The model under review builds one solid part; all positions refer to its coordinate system, in mm. A direction names the side the tool comes from. Coordinates: 2 decimals unless noted, no trailing zeros. Loops run counter-clockwise (first coordinate to the right, second up) from the corner with the lowest first, then second, coordinate; pieces in that order, holes last. Notation, with made-up numbers: (-34, -12.5) - (23, -12.5) arc R13 ccw to (23, -7.5) - close; hole circle Ø1 at (75.25, -3.5). An arc over 180 degrees is marked (long way). Answer in a Markdown table with one row per item. Add a question column.
(1) We need section A-A on x = -38.1. Write out the cut boundary in (y, z), plus the area to 3 significant figures.
(2) We need section B-B on y = 12.7. Write out the cut boundary in (x, z), plus the area to 3 significant figures.
(3) We need section C-C on y = 0. Give the number of separate pieces and of enclosed holes in the cut face, plus the area to 3 significant figures.
(4) For P1, Ø0.8, axis at y = -16.5, z = 0.5, coming from the +X side; P2, Ø2.5, axis at x = -62.5, y = -2, coming from the +Z side; P3, Ø0.6, axis at x = -65.5, z = 0, coming from the -Y side; P4, Ø0.8, axis at y = -7.5, z = 0, coming from the +X side, all flat-tipped, find the tip position at first contact; note any pin that passes through.
(5) Mouldability with a two-part tool opening along Y and no side actions: class faces 3 (the flat face through (-1, 38.1, 9)), 4 (the flat face through (-1, -38.1, 9)), 5 (the cylindrical face through (63, -15.293, 1.198)) as +Y half, -Y half, draft (parallel to the pull), parting line (faces both ways), or undercut.
(6) For line 1 along X through (y, z) = (-12.7, 13.75); line 2 along X through (y, z) = (11, 8.75); line 3 along Y through (x, z) = (63.5, 9.25), list the stretches that pass through material, from the lowest coordinate up.
(7) Machinability: for faces 1 (the cylindrical face through (58.25, -15.04, 9.46)), 2 (the flat face through (68.67, -31.66, 8.96)), which of the approach directions +Z, -Z, +X, -X, +Y, -Y give a long, thin tool a straight path to every point of the face, cutting with its end or side? Answer none if there is none.
from build123d import *

# Parameters (mm, degrees)
SKETCH1_W                                    = 149.86
SKETCH1_H                                    = 76.2
EXTRUDE1_DEPTH                               = 17.399
SKETCH2_W                                    = 149.86
SKETCH2_H                                    = 76.2
SKETCH2_W_2                                  = 19.05
SKETCH2_H_2                                  = 38.1
CUT_EXTRUDE1_DEPTH                           = 0.762
F_10_32_TAPPED_HOLE1_D                       = 4.0386
CBORE_FOR_10_SOCKET_HEAD_CAP_SCREW1_AT_COUNT = 2
CBORE_FOR_10_SOCKET_HEAD_CAP_SCREW1_AT_PITCH = 25.4
CBORE_FOR_10_SOCKET_HEAD_CAP_SCREW1_2_COUNT  = 2
CBORE_FOR_10_SOCKET_HEAD_CAP_SCREW1_2_PITCH  = 124.499845703
CHAMFER1_SIZE                                = 12.7
SKETCH7_W                                    = 1.5748
SKETCH7_H                                    = 38.1
CUT_EXTRUDE2_DEPTH                           = 0.762
F_13_32_0_40625_DIAMETER_HOLE1_D             = 10.31875


with BuildPart() as part:
    # Sketch1 → Extrude1 (new body)
    with BuildSketch(Plane.XY):
        Rectangle(SKETCH1_W, SKETCH1_H)
    extrude(amount=EXTRUDE1_DEPTH)

    # Sketch2 → Cut-Extrude1 (cut)
    with BuildSketch(Plane(origin=(0, 0, 0), x_dir=(-1, 0, 0), z_dir=(0, 0, -1))):
        Rectangle(SKETCH2_W, SKETCH2_H)
        with Locations((-61.9252, 0)):
            Rectangle(SKETCH2_W_2, SKETCH2_H_2, mode=Mode.SUBTRACT)
        with Locations((61.9252, 0)):
            Rectangle(SKETCH2_W_2, SKETCH2_H_2, mode=Mode.SUBTRACT)
    extrude(amount=-CUT_EXTRUDE1_DEPTH, mode=Mode.SUBTRACT)

    # #10-32 Tapped Hole1 (through all)
    with Locations(Plane.XY.offset(17.399)):
        with Locations((61.9252, 0), (-61.9252, -12.7), (-61.9252, 12.7)):
            Hole(F_10_32_TAPPED_HOLE1_D / 2)

    # Sketch5 → CBORE for #10 Socket Head Cap Screw1 (revolve, cut)
    with BuildSketch(Plane(origin=(61.9252, -12.7, 17.399), x_dir=(0, -1, 0), z_dir=(1, 0, 0))):
        Polygon((0, 0), (0, 17.399), (2.8067, 17.399), (2.8067, 15.0368), (4.3561, 15.0368), (4.3561, 1.0414), (5.3975, 0), align=None)
    cbore_for_10_socket_head_cap_screw1 = revolve(axis=Axis((61.9252, -12.7, 23.749), (0, 0, -1)), mode=Mode.SUBTRACT)

    # CBORE for #10 Socket Head Cap Screw1 at: CBORE for #10 Socket Head Cap Screw1 ×2
    with Locations(*[(0, i * CBORE_FOR_10_SOCKET_HEAD_CAP_SCREW1_AT_PITCH, 0) for i in range(1, CBORE_FOR_10_SOCKET_HEAD_CAP_SCREW1_AT_COUNT)]):
        add(cbore_for_10_socket_head_cap_screw1, mode=Mode.SUBTRACT)

    # CBORE for _10 Socket Head Cap Screw1 2: CBORE for #10 Socket Head Cap Screw1 ×2
    with Locations(*[Vector(-0.994783562, 0.102008159, 0) * (i * CBORE_FOR_10_SOCKET_HEAD_CAP_SCREW1_2_PITCH) for i in range(1, CBORE_FOR_10_SOCKET_HEAD_CAP_SCREW1_2_COUNT)]):
        add(cbore_for_10_socket_head_cap_screw1, mode=Mode.SUBTRACT)

    # Chamfer1
    chamfer1_edges = [part.edges().sort_by_distance(p)[0] for p in [
        (74.93, -38.1, 9.0805),
        (-74.93, -38.1, 9.0805),
        (-74.93, 38.1, 9.0805),
        (74.93, 38.1, 9.0805),
    ]]
    chamfer(chamfer1_edges, length=CHAMFER1_SIZE)

    # Sketch7 → Cut-Extrude2 (cut)
    with BuildSketch(Plane(origin=(0, 0, 0), x_dir=(-1, 0, 0), z_dir=(0, 0, -1))):
        with Locations((61.9252, 0)):
            Rectangle(SKETCH7_W, SKETCH7_H)
        with Locations((-61.9252, 0)):
            Rectangle(SKETCH7_W, SKETCH7_H)
    extrude(amount=-CUT_EXTRUDE2_DEPTH, mode=Mode.SUBTRACT)

    # 13/32 (0.40625) Diameter Hole1 (through all)
    with Locations(Plane.XY.offset(17.399)):
        with Locations((-38.1, 0), (38.1, 0)):
            Hole(F_13_32_0_40625_DIAMETER_HOLE1_D / 2)


solid = part.part
Outcome:
| question | item | result |
|---|---|---|
| 1 | outline | (-38.1, 0.76) - (-5.16, 0.76) - (-5.16, 17.4) - (-38.1, 17.4) - close; (5.16, 0.76) - (38.1, 0.76) - (38.1, 17.4) - (5.16, 17.4) - close |
| 1 | area | 1,100 mm² |
| 2 | outline | (-74.93, 0.76) - (-71.45, 0.76) - (-71.45, 0) - (-63.94, 0) - (-63.94, 17.4) - (-74.93, 17.4) - close; (-59.91, 0) - (-52.4, 0) - (-52.4, 0.76) - (52.4, 0.76) - (52.4, 0) - (59.12, 0) - (59.12, 2.36) - (57.57, 2.36) - (57.57, 16.36) - (56.53, 17.4) - (-59.91, 17.4) - close; (64.73, 0) - (71.45, 0) - (71.45, 0.76) - (74.93, 0.76) - (74.93, 17.4) - (67.32, 17.4) - (66.28, 16.36) - (66.28, 2.36) - (64.73, 2.36) - close |
| 2 | area | 2,310 mm² |
| 3 | separate pieces | 5 |
| 3 | enclosed holes | 0 |
| 3 | area | 1,960 mm² |
| 4 | P1 | x = 74.93 |
| 4 | P2 | z = 2.36 |
| 4 | P3 | y = -19.05 |
| 4 | P4 | x = 71.45 |
| 5 | face 3 | +Y half |
| 5 | face 4 | -Y half |
| 5 | face 5 | undercut |
| 6 | line 1 | -74.93 to -63.94, -59.91 to 57.57, 66.28 to 74.93 |
| 6 | line 2 | -74.93 to -63.01, -60.84 to 57.91, 65.94 to 74.93 |
| 6 | line 3 | -36.83 to -16.76, -8.64 to -1.26, 1.26 to 8.64, 16.76 to 36.83 |
| 7 | face 1 | +Z |
| 7 | face 2 | +Z, -Z, +X, -Y |
